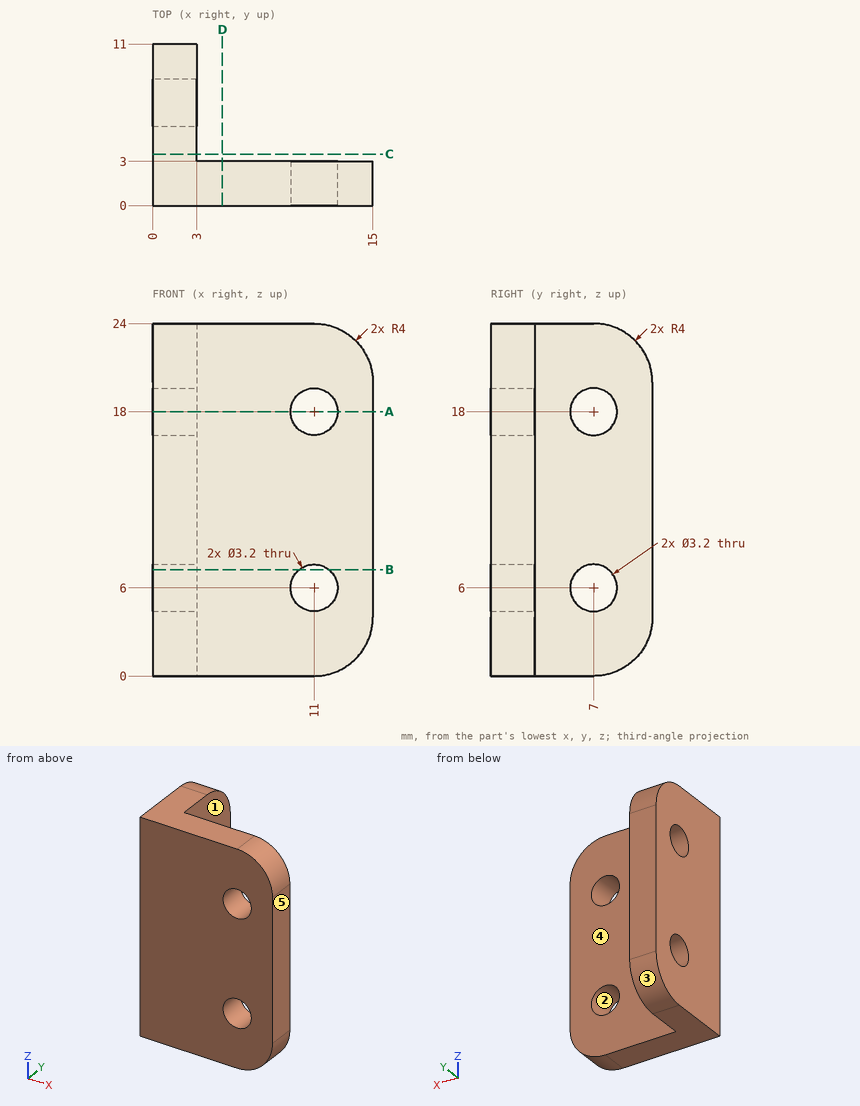
Verification items for this drawing (mm, ordinates from the low corner). A direction names the side the tool comes from. Give positions to 0.01 mm unless a question says otherwise; leave off trailing zeros. Loops run counter-clockwise (first coordinate to the right, second up) from the corner with the lowest first, then second, coordinate; pieces in that order, holes last. Notation, with made-up numbers: (-3, 27.5) - (45, 27.5) arc R24 cw to (45, 46.5) - close; hole circle Ø9 at (76, 46.5). An arc over 180 degrees is marked (long way). Write item = value, one per line. Start each with the question number.
Q1. Depth check by flat-ended pin: P1, Ø3, axis at x = 8, y = 6, coming from the -Z side; P2, Ø1.5, axis at y = 9.5, z = 7.5, coming from the +X side; P3, Ø2, axis at x = 13.5, z = 8.5, coming from the +Y side. Enter the tip coordinate at first touch or a pass-through.
Q2. Thickness scan on line 1 (Z direction, x = 2.4, y = 7); line 2 (X direction, y = 10.5, z = 13.5). Record the ranges inside material, lowest first.
Q3. Mould release check, pull along X, two halves, no side actions. Record for the marked faces 1, 2 and 3: released by +X, released by -X, zero draft, split by the parting line, or undercut.
Q4. Cross-section at B-B, the plane z = 7.25. Enter the section's corners in (x, y).
Q5. Tool access check on the marked faces 4 and 5. Record the directions out of +Z, -Z, +X, -X, +Y, -Y that give a thin tool (end or side, any length) a straight path to the whole face; none if there is none.
Q6. Cross-section at A-A, the plane z = 18. Enter the section's corners in (x, y).
Q7. Cross-section at C-C, the plane y = 3.5. Enter the section's corners in (x, z), and give its area (3 significant figures).
Answer key:
q1.P1 = through
q1.P2 = 3
q1.P3 = 3
q2.line_1 = 0 to 4.4, 7.6 to 16.4, 19.6 to 24
q2.line_2 = 0 to 3
q3.face_1 = released by +X
q3.face_2 = undercut
q3.face_3 = zero draft
q4.outline = (0, 0) - (10, 0) - (10, 3) - (3, 3) - (3, 6) - (0, 6) - close; (0, 8) - (3, 8) - (3, 11) - (0, 11) - close; (12, 0) - (15, 0) - (15, 3) - (12, 3) - close
q5.face_4 = +Z, -Z, +X, +Y
q5.face_5 = +Z, -Z, +X, +Y, -Y
q6.outline = (0, 0) - (9.4, 0) - (9.4, 3) - (3, 3) - (3, 5.4) - (0, 5.4) - close; (0, 8.6) - (3, 8.6) - (3, 11) - (0, 11) - close; (12.6, 0) - (15, 0) - (15, 3) - (12.6, 3) - close
q7.outline = (0, 0) - (3, 0) - (3, 24) - (0, 24) - close
q7.area = 72.0 mm^2
